Autodesk Inventor part; units mm, degrees
ref_plane "YZ Plane" through (0, 0, 0) normal (1, 0, 0) x (0, 1, 0)
ref_plane "XZ Plane" through (0, 0, 0) normal (0, 1, 0) x (-1, 0, 0)
ref_plane "XY Plane" through (0, 0, 0) normal (0, 0, 1) x (1, 0, 0)
sketch "Náčrt1" plane through (0, 0, 0) normal (0, 0, 1) x (1, 0, 0)
  circle A0 centre (0, 0) radius 24.5
  dimension "d0" = 49
extrude "Vysunutí1" add sketch "Náčrt1" along normal mid plane 10
sketch "Náčrt2" plane through (0, 0, 5) normal (0, 0, 1) x (1, 0, 0)
  circle A0 centre (0, 0) radius 20
  dimension "d3" = 40
extrude "Vysunutí2" add sketch "Náčrt2" along normal blind 18
sketch "Náčrt3" plane through (0, 0, -5) normal (0, 0, -1) x (-1, 0, 0)
  circle A0 centre (0, 0) radius 21
  dimension "d6" = 42
extrude "Vysunutí3" add sketch "Náčrt3" along normal blind 48
sketch "Náčrt4" plane through (0, 0, -53) normal (0, 0, -1) x (-1, 0, 0)
  circle A0 centre (0, 0) radius 20
  dimension "d9" = 40
extrude "Vysunutí4" add sketch "Náčrt4" along normal blind 48
sketch "Náčrt5" plane through (0, 0, -101) normal (0, 0, -1) x (-1, 0, 0)
  circle A0 centre (0, 0) radius 16
  dimension "d12" = 32
extrude "Vysunutí5" add sketch "Náčrt5" along normal blind 58
sketch "Náčrt6" plane through (0, 0, 0) normal (1, 0, 0) x (0, 1, 0)
  line L0 (0, -9) -> (0, -49) construction
  line L1 (-6, -15) -> (-6, -43)
  line L2 (6, -43) -> (6, -15)
  arc A0 (6, -15) -> (-6, -15) centre (0, -15) ccw
  arc A1 (-6, -43) -> (6, -43) centre (0, -43) ccw
  line L3 (-24.5, -5) -> (24.5, -5)
  line L4 (0, -195.4) -> (0, 59.4)
  line L5 (-21, -53) -> (21, -53)
  point P0 (0, 0)
  point P1 (0, -29)
  dimension "d15" = 12
  dimension "d16" = 4
  dimension "d17" = 4
extrude "Vysunutí6" cut sketch "Náčrt6" along normal through all
sketch "Náčrt7" plane through (0, 0, 0) normal (1, 0, 0) x (0, 0, -1)
  line L0 (15, -6) -> (43, -6)
  arc A0 (43, -6) -> (43, 6) centre (43, 0) ccw
  line L1 (43, 6) -> (15, 6)
  arc A1 (15, 6) -> (15, -6) centre (15, 0) ccw
  point P0 (0, 0)
extrude "Vysunutí7" add sketch "Náčrt7" along normal blind 16.1 and the other way blind 18.55
sketch "Náčrt8" plane through (0, 0, 0) normal (1, 0, 0) x (0, 1, 0)
  line L0 (0, -195.4) -> (0, 59.4)
  line L1 (0, -106) -> (0, -151) construction
  line L2 (-5, -111) -> (-5, -146)
  line L3 (5, -146) -> (5, -111)
  arc A0 (5, -111) -> (-5, -111) centre (0, -111) ccw
  arc A1 (-5, -146) -> (5, -146) centre (0, -146) ccw
  line L4 (-20, -101) -> (20, -101)
  point P0 (0, 0)
  point P1 (0, -128.5)
  dimension "d24" = 10
  dimension "d25" = 5
  dimension "d26" = 35
extrude "Vysunutí8" cut sketch "Náčrt8" along normal through all
sketch "Náčrt9" plane through (0, 0, 0) normal (1, 0, 0) x (0, 0, -1)
  line L0 (111, -5) -> (146, -5)
  arc A0 (146, -5) -> (146, 5) centre (146, 0) ccw
  line L1 (146, 5) -> (111, 5)
  arc A1 (111, 5) -> (111, -5) centre (111, 0) ccw
  point P0 (0, 0)
extrude "Vysunutí9" add sketch "Náčrt9" along normal blind 11.3
chamfer "Zkosení1" distance 1 angle 45 1 edges at (-20, 0, 23)
fillet "Zaoblení2" radius 1 3 edges at (21, 0, -5) (20, 0, -53) (16, 0, -159)
fillet "Zaoblení2" radius 2.5 1 edges at (16, 0, -101)
properties part number "hridel"
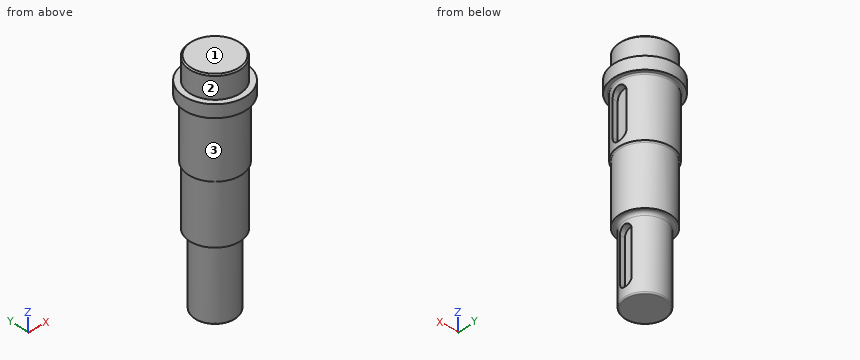
CAD build for the part. Positions are in the model's coordinates, mm. Face numbers are marked on the shaded views. A direction names the side the tool comes from. Round coordinates to 2 decimals unless told otherwise and drop trailing zeros. Order: outer loops, then holes, each group sorted by start corner. A loop starts at its lowest first (then second) coordinate and runs counter-clockwise, first axis right, second up. Notation, with made-up numbers: (-1.5, -5.5) - (40.5, -5.5) arc R23 cw to (40.5, 20.5) - close; hole circle Ø6 at (3.5, -11.75). An arc over 180 degrees is marked (long way). Return JSON: item names as keys, results as strings.
(1) Cut at B-B (z = -138.5). Give the cut face in (x, y).
Answer key:
{"outline": "(11.3, -5) - (11.3, 5) - (15.2, 5) arc R16 ccw (long way) to (15.2, -5) - close"}
(2) Cut at D-D (z = -29.5). Give the cut face in (x, y), then the cut area to 3 significant figures.
Answer key:
{"outline": "(16.1, -6) - (16.1, 6) - (20.12, 6) arc R21 ccw (long way) to (20.12, -6) - close", "area": "1,330 mm^2"}
(3) Wall check: probe 1 along Y at (x, z) = (0.5, -109); probe 2 along Z at (x, y) = (-19, 12.5); probe 3 along X at (y, z) = (1, -141). Give the ranges that are in metal, low to high. Write a range as from..to.
Answer key:
{"probe 1": "y = -15.99..15.99", "probe 2": "z = -5..5", "probe 3": "x = -15.97..11.3"}
(4) Cut at C-C (z = -90). Give the cut face in (x, y).
Answer key:
{"outline": "circle Ø40 at (0, 0)"}
(5) Pin check, flat tips, straight feed: pin 1 Ø3 at (x, y) = (-15.5, 13) entering from -Z; pin 2 Ø3 at (y, z) = (2, -129) entering from +X; pin 3 Ø4.5 at (x, z) = (13, -124.5) entering from -Y; pin 4 Ø5 at (x, y) = (-11.5, -11) entering from -Z. Stop position of each tip, or through.
Answer key:
{"pin 1": "stops at z = -101", "pin 2": "stops at x = 11.3", "pin 3": "stops at y = -11.85", "pin 4": "stops at z = -159"}
(6) Tool access for the marked faces 1, 2 and 3: list every direction of +Z, -Z, +X, -X, +Y, -Y with a clear straight run to the whole face (end or side of a thin tool).
Answer key:
{"face 1": "+Z, +X, -X, +Y, -Y", "face 2": "+Z", "face 3": "-Z"}
